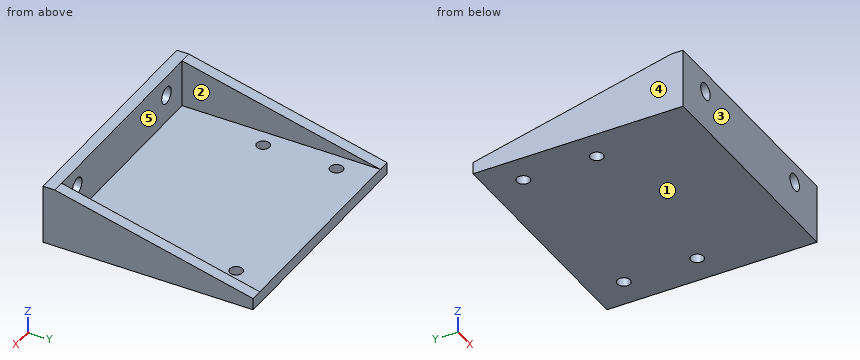
```python
from build123d import *

# Parameters (mm, degrees)
SKETCH1_W           = 60
SKETCH1_H           = 15
SKETCH1_R           = 2.125
BOSS_EXTRUDE1_DEPTH = 3
SKETCH2_W           = 60
SKETCH2_H           = 50
SKETCH2_R           = 1.625
BOSS_EXTRUDE2_DEPTH = 3
BOSS_EXTRUDE3_DEPTH = 3


with BuildPart() as part:
    # Sketch1 → Boss-Extrude1 (new body)
    with BuildSketch(Plane(origin=(0, 0, 0), x_dir=(1, 0, 0), z_dir=(0, 1, 0))):
        with Locations((30, 7.5)):
            Rectangle(SKETCH1_W, SKETCH1_H)
        with Locations(Location((10, 5, 0), (0, 0, 270))):
            Circle(SKETCH1_R, mode=Mode.SUBTRACT)
        with Locations(Location((50, 5, 0), (0, 0, 90))):
            Circle(SKETCH1_R, mode=Mode.SUBTRACT)
    extrude(amount=BOSS_EXTRUDE1_DEPTH)

    # Sketch2 → Boss-Extrude2 (add)
    with BuildSketch(Plane(origin=(0, 0, -15), x_dir=(-1, 0, 0), z_dir=(0, 0, -1))):
        with Locations((-30, 28)):
            Rectangle(SKETCH2_W, SKETCH2_H)
        with Locations((-52.5, 44.5)):
            Circle(SKETCH2_R, mode=Mode.SUBTRACT)
        with Locations((-52.5, 26)):
            Circle(SKETCH2_R, mode=Mode.SUBTRACT)
        with Locations(Location((-7.5, 26, 0), (0, 0, 180))):
            Circle(SKETCH2_R, mode=Mode.SUBTRACT)
        with Locations(Location((-7.5, 44.5, 0), (0, 0, 180))):
            Circle(SKETCH2_R, mode=Mode.SUBTRACT)
    extrude(amount=-BOSS_EXTRUDE2_DEPTH)

    # Sketch3 → Boss-Extrude3 (add)
    with BuildSketch(Plane.ZY):
        Polygon((-12, 53), (0, 3), (-12, 3), align=None)
    boss_extrude3 = extrude(amount=-BOSS_EXTRUDE3_DEPTH)

    # Mirror1: Boss-Extrude3 across plane
    add(boss_extrude3.mirror(Plane.ZY.offset(-30)))


solid = part.part
```
The model under review builds one solid part; all positions refer to its coordinate system, in mm. Face numbers are marked on the shaded views. A direction names the side the tool comes from. Coordinates: 2 decimals unless noted, no trailing zeros. Write each loop counter-clockwise with the first axis right and the second up, starting at its lowest first coordinate (ties: lowest second). Pieces come first, ordered by that corner, then holes. Notation, with made-up numbers: (7, 14.25) - (53, 14.25) arc R13 cw to (53, 28.25) - close; hole circle Ø9 at (37, 14). An arc over 180 degrees is marked (long way). Write item = value, one per line.
(1) Mouldability with a two-part tool opening along X and no side actions: class the marked faces 3, 4 and 5 as pulls with the +X half, pulls with the -X half, needs draft (parallel to the pull), parting line crosses it, or undercut.
Result sheet:
face_3 = needs draft
face_4 = pulls with the -X half
face_5 = undercut
(2) Consider section C-C, the plane y = 32. Give the boundary of the cut face in (x, z).
Result sheet:
outline = (0, -15) - (60, -15) - (60, -6.96) - (57, -6.96) - (57, -12) - (3, -12) - (3, -6.96) - (0, -6.96) - close
(3) For line 1 (Y direction, x = 52.5, z = -13.55) (3 decimals); line 2 (X direction, y = 20, z = -6.5); line 3 (Z direction, x = 52, y = 11), list the stretches that pass through material, from the lowest coordinate up. Write a range as [from, to].
Result sheet:
line_1 = [0, 24.375], [27.625, 42.875], [46.125, 53]
line_2 = [0, 3], [57, 60]
line_3 = [-15, -12]
(4) Machinability: for the marked faces 1 and 2, which of the approach directions +Z, -Z, +X, -X, +Y, -Y give a long, thin tool a straight path to every point of the face, cutting with its end or side? Answer none if there is none.
Result sheet:
face_1 = -Z, +X, -X, +Y, -Y
face_2 = +Z, +Y
(5) Consider section B-B, the plane z = -5. Give the boundary of the cut face in (x, y) (3 decimals), then the cut area to 4 significant figures.
Result sheet:
outline = (0, 0) - (7.875, 0) - (7.875, 3) - (3, 3) - (3, 23.833) - (0, 23.833) - close; (12.125, 0) - (47.875, 0) - (47.875, 3) - (12.125, 3) - close; (52.125, 0) - (60, 0) - (60, 23.833) - (57, 23.833) - (57, 3) - (52.125, 3) - close
area = 279.5 mm^2
(6) Consider section A-A, the plane y = 26. Give the boundary of the cut face in (x, z) (3 decimals).
Result sheet:
outline = (0, -15) - (5.875, -15) - (5.875, -12) - (3, -12) - (3, -5.52) - (0, -5.52) - close; (9.125, -15) - (50.875, -15) - (50.875, -12) - (9.125, -12) - close; (54.125, -15) - (60, -15) - (60, -5.52) - (57, -5.52) - (57, -12) - (54.125, -12) - close
(7) For P1, Ø2, axis at x = 29.5, y = 39, coming from the +Z side; P2, Ø5, axis at x = 8.5, z = -9, coming from the +Y side, all flat-tipped, find the tip position at first contact; note any pin that passes through.
Result sheet:
P1 = -12
P2 = 3
(8) Consider section D-D, the plane x = 29.5. Give the boundary of the cut face in (y, z).
Result sheet:
outline = (0, -15) - (53, -15) - (53, -12) - (3, -12) - (3, 0) - (0, 0) - close
